```python
from build123d import *

# Parameters (mm, degrees)
CROQUIS1_R                 = 1.6
SALIENTE_EXTRUIR1_DEPTH    = 3.5
CORTAR_EXTRUIR1_DEPTH      = 14.910427743
CORTAR_EXTRUIR1_DEPTH_BACK = 14.910427743
CROQUIS2_R                 = 1.5
REDONDEO1_R                = 1
REDONDEO2_R                = 0.5


with BuildPart() as part:
    # Croquis1 → Saliente-Extruir1 (new, symmetric)
    with BuildSketch(Plane.XY):
        with BuildLine():
            Line((3, 11.5), (7, 11.5))
            Line((7, 11.5), (7, -6.5))
            Line((7, -6.5), (4.9, -6.5))
            ThreePointArc((4.9, -6.5), (3.4, -8), (4.9, -9.5))
            Line((4.9, -9.5), (7, -9.5))
            Line((7, -9.5), (7, -11.5))
            Line((7, -11.5), (-7, -11.5))
            Line((-7, -11.5), (-7, -9.5))
            Line((-7, -9.5), (-4.9, -9.5))
            ThreePointArc((-4.9, -9.5), (-3.4, -8), (-4.9, -6.5))
            Line((-4.9, -6.5), (-7, -6.5))
            Line((-7, -6.5), (-7, 11.5))
            Line((-7, 11.5), (-3, 11.5))
            Line((-3, 11.5), (-3, 3.5))
            Line((-3, 3.5), (3, 3.5))
            Line((3, 3.5), (3, 11.5))
        make_face()
        with Locations((0, -4)):
            Circle(CROQUIS1_R, mode=Mode.SUBTRACT)
    extrude(amount=SALIENTE_EXTRUIR1_DEPTH, both=True)

    # Croquis2 → Cortar-Extruir1 (cut, two sides: drawn at the far end of the back side and taken through both)
    with BuildSketch(Plane(origin=(0, 0, 0), x_dir=(0, 0, -1), z_dir=(1, 0, 0)).offset(-CORTAR_EXTRUIR1_DEPTH_BACK)):
        with Locations((0, 7.5)):
            Circle(CROQUIS2_R)
    extrude(amount=CORTAR_EXTRUIR1_DEPTH + CORTAR_EXTRUIR1_DEPTH_BACK, mode=Mode.SUBTRACT)

    # Redondeo1
    redondeo1_edges = [part.edges().sort_by_distance(p)[0] for p in [
        (-7, 11.5, 0),
        (-3, 11.5, 0),
        (-3, 3.5, 0),
        (3, 3.5, 0),
        (3, 11.5, 0),
        (7, 11.5, 0),
    ]]
    fillet(redondeo1_edges, radius=REDONDEO1_R)

    # Redondeo2
    redondeo2_edges = [part.edges().sort_by_distance(p)[0] for p in [
        (7, -11.5, 0),
        (-7, -11.5, 0),
        (-7, -9.5, 0),
        (-7, -6.5, 0),
        (7, -6.5, 0),
        (7, -9.5, 0),
    ]]
    fillet(redondeo2_edges, radius=REDONDEO2_R)


solid = part.part
```
Design review of the part built by this model. Coordinates are the model's own, in mm. A direction names the side the tool comes from. Round coordinates to 2 decimals unless told otherwise and drop trailing zeros. Write each loop counter-clockwise with the first axis right and the second up, starting at its lowest first coordinate (ties: lowest second). Pieces come first, ordered by that corner, then holes.
Item 1: We need section B-B on y = 7.5. Write out the cut boundary in (x, z).
Item 2: Clearance check with a flat-ended pin moving along its axis: pin 1 Ø1.8 at (y, z) = (7.5, 0) entering from +X. State where the tip first meets the part, or that it passes through.
Item 3: For probe 1 along Y at (x, z) = (5.7, 0); probe 2 along Z at (x, y) = (-5.1, 7.5); probe 3 along Y at (x, z) = (0, 0.5), list the stretches that pass through material, from the lowest coordinate up.
Item 4: The part is to be moulded in two halves that separate along Z. For faces 6 (the flat face through (0, 0, 3.5)), 7 (the flat face through (7, 2, 0)), 8 (the cylindrical face through (-5, 6, 0)), 9 (the cylindrical face through (5, 6, 0)), say which applies: +Z half, -Z half, draft (parallel to the pull), parting line (faces both ways), or undercut.
Item 5: For faces 1 (the flat face through (-6, -9.5, 0)), 2 (the flat face through (5, 11.5, 0)), 3 (the flat face through (0, -11.5, 0)), 4 (the cylindrical face through (2.715, 3.801, 0.049)), 5 (the flat face through (6, -6.5, 0)), list the 3-axis set-ups (+Z, -Z, +X, -X, +Y, -Y) from which the entire face can be reached by the end or side of a thin tool; tool diameter is ignored.
Item 6: We need section C-C on x = 0. Write out the cut boundary in (y, z).
Item 7: We need section A-A on y = -4. Write out the cut boundary in (x, z), and give its area (3 significant figures).
Returned:
1. outline: (-7, -3.5) - (-3, -3.5) - (-3, -1.5) - (-7, -1.5) - close; (-7, 1.5) - (-3, 1.5) - (-3, 3.5) - (-7, 3.5) - close; (3, -3.5) - (7, -3.5) - (7, -1.5) - (3, -1.5) - close; (3, 1.5) - (7, 1.5) - (7, 3.5) - (3, 3.5) - close
2. pin 1: passes through
3. probe 1: y = -11.5 to -9.5, -6.5 to 6, 9 to 11.5
3. probe 2: z = -3.5 to -1.5, 1.5 to 3.5
3. probe 3: y = -11.5 to -5.6, -2.4 to 3.5
4. face 6: +Z half
4. face 7: draft
4. face 8: undercut
4. face 9: undercut
5. face 1: +Z, -Z, -X
5. face 2: +Z, -Z, +X, -X, +Y
5. face 3: +Z, -Z, +X, -X, -Y
5. face 4: +Z, -Z, +Y
5. face 5: +Z, -Z, +X
6. outline: (-11.5, -3.5) - (-5.6, -3.5) - (-5.6, 3.5) - (-11.5, 3.5) - close; (-2.4, -3.5) - (3.5, -3.5) - (3.5, 3.5) - (-2.4, 3.5) - close
7. outline: (-7, -3.5) - (-1.6, -3.5) - (-1.6, 3.5) - (-7, 3.5) - close; (1.6, -3.5) - (7, -3.5) - (7, 3.5) - (1.6, 3.5) - close
7. area: 75.6 mm2
